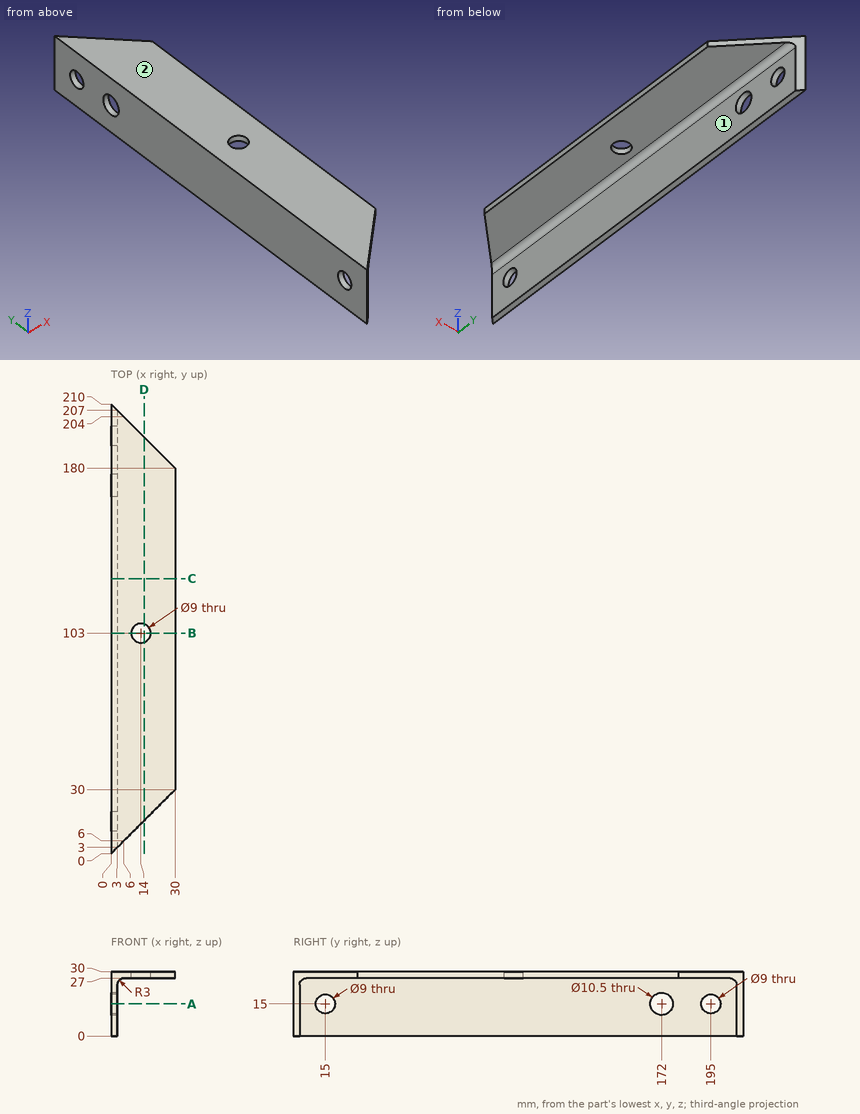
The drawing under review shows one solid part. Ordinate dimensions are in mm from its lowest x, y, z. A direction names the side the tool comes from. Coordinates: 2 decimals unless noted, no trailing zeros. Order: outer loops, then holes, each group sorted by start corner. A loop starts at its lowest first (then second) coordinate and runs counter-clockwise, first axis right, second up. Notation, with made-up numbers: M 19,71.25 L 72,71.25 A25 cw 72,91.25 Z; hole C -9,-3.5 d8. An arc over 180 degrees is marked long. One line per question, with ' | ' between items.
(1) Add section D-D, the plane x = 15.5. Write out the cut boundary in (y, z).
Geometry results:
outline: M 15.5,27 L 98.76,27 L 98.76,30 L 15.5,30 Z; M 107.24,27 L 194.5,27 L 194.5,30 L 107.24,30 Z
(2) For probe 1 along Z at (x, y) = (0.6, 15); probe 2 along X at (y, z) = (23, 7.5); probe 3 along Z at (x, y) = (13, 143), list the stretches that pass through material, from the lowest coordinate up. Write a range as from..to.
Geometry results:
probe 1: z = 0..10.5, 19.5..30 | probe 2: x = 0..3 | probe 3: z = 27..30
(3) Machinability: for the marked faces 1 and 2, which of the approach directions +Z, -Z, +X, -X, +Y, -Y give a long, thin tool a straight path to every point of the face, cutting with its end or side? Answer none if there is none.
Geometry results:
face 1: -Z, +X, +Y, -Y | face 2: +Z, +X, -X, +Y, -Y
(4) Add section A-A, the plane z = 15. Write out the cut boundary in (x, y), then the cut area to 4 significant figures.
Geometry results:
outline: M 0,0 L 3,3 L 3,10.5 L 0,10.5 Z; M 0,19.5 L 3,19.5 L 3,166.75 L 0,166.75 Z; M 0,177.25 L 3,177.25 L 3,190.5 L 0,190.5 Z; M 0,199.5 L 3,199.5 L 3,207 L 0,210 Z | area: 535.5 mm²
(5) Add section C-C, the plane y = 128.5. Write out the cut boundary in (x, z).
Geometry results:
outline: M 0,0 L 3,0 L 3,24 A3 cw 6,27 L 30,27 L 30,30 L 0,30 Z
(6) Add section B-B, the plane y = 103. Write out the cut boundary in (x, z), then the cut area to 3 significant figures.
Geometry results:
outline: M 0,0 L 3,0 L 3,24 A3 cw 6,27 L 9.5,27 L 9.5,30 L 0,30 Z; M 18.5,27 L 30,27 L 30,30 L 18.5,30 Z | area: 146 mm²
(7) Insertion check: pin 1 (4 mm diameter, centred on y = 84, z = 22.5, fed in from +X); pin 2 (12 mm diameter, centred on x = 17.5, y = 144.5, fed in from -Z); pin 3 (1 mm diameter, centred on x = 4.5, y = 176, fed in from -Z). Each pin has a flat end and moves straight along its axis. Give the tip position at first contact, or say it passes through.
Geometry results:
pin 1: stops at x = 3.04 | pin 2: stops at z = 27 | pin 3: stops at z = 26.24
